Design review of the part built by this model. Coordinates are the model's own, in mm. A direction names the side the tool comes from. Round coordinates to 2 decimals unless told otherwise and drop trailing zeros. Loops run counter-clockwise (first coordinate to the right, second up) from the corner with the lowest first, then second, coordinate; pieces in that order, holes last. Notation, with made-up numbers: (51.25, -24) - (60.25, -24) arc R12 cw to (60.25, -6) - close; hole circle Ø2 at (25, 34.25). An arc over 180 degrees is marked (long way). Answer as CSV lines item,"result". Start each with the question number.
(1) Consider section B-B (y = 0). Count the separate pieces of the cut face and the enclosed holes in it, and give its area (3 significant figures).
(2) For P1, Ø1, axis at x = 140.5, z = 4.5, coming from the -Y side; P2, Ø12, axis at x = 28.5, y = 2, coming from the -Z side; P3, Ø6, axis at y = 10, z = -6, coming from the -X side, all flat-tipped, find the tip position at first contact; note any pin that passes through.
(3) Consider section C-C (z = 22). Give the boundary of the cut face in (x, y).
(4) Consider section A-A (x = 0). Give the boundary of the cut face in (y, z), and give its area (3 significant figures).
(5) For faces 3 (the flat face through (-3, -5.4, 0)), 4 (the cylindrical face through (132.387, 7.154, 2.253)), 5 (the flat face through (-3, -5.4, 25)), list the 3-axis set-ups (+Z, -Z, +X, -X, +Y, -Y) from which the entire face can be reached by the end or side of a thin tool; tool diameter is ignored.
(6) Mouldability with a two-part tool opening along X and no side actions: class faces 1 (the cylindrical face through (161.923, 3.755, 0.175)), 2 (the flat face through (155.4, 3, 12.5)) as released by +X, released by -X, zero draft, split by the parting line, or undercut.
(7) Wall thickness on L1, parallel to Y at x = 150, z = 0; L2, parallel to Z at x = -4.5, y = -8; L3, parallel to Y at x = 51, z = 9: over which ranges is each line inside the solid? List them lowest first.
from build123d import *

# Parameters (mm, degrees)
F0_R      = 12.5
F0_R_2    = 6
F1_DEPTH  = 25
F3_R      = 12.5
F3_R_2    = 6
F4_DEPTH  = 12.5
F5_R      = 7.5
F7_R      = 6
F8_DEPTH  = 25
F9_R      = 6
F10_DEPTH = 25


# Not quite as in the source:
# - a feature names something its author has since deleted; it is built from what else it names


with BuildPart() as f1:
    # F0 (on Top) → F1 (new body)
    with BuildSketch(Plane.XY):
        Circle(F0_R)
        Circle(F0_R_2, mode=Mode.SUBTRACT)
    extrude(amount=F1_DEPTH)



with BuildPart() as f4:
    # F3 (on Top) → F4 (new body, symmetric)
    with BuildSketch(Plane.XY):
        with Locations((150, 0)):
            Circle(F3_R)
        with Locations((150, 0)):
            Circle(F3_R_2, mode=Mode.SUBTRACT)
    extrude(amount=F4_DEPTH, both=True)


with BuildPart() as f1_1:
    add(f1.part)

    add(f4.part)  # F6 merges F4
    # F6: sweep along a path in F2
    with BuildLine(Plane.XZ) as f6_path:
        Line((0, 12.5), (25, 12.5))
        ThreePointArc((25, 12.5), (33.2790451747, 11.9260667636), (41.399703043, 10.2152470332))
        Line((41.399703043, 10.2152470332), (64.3324330449, 6.6001820378))
        Line((64.3324330449, 6.6001820378), (81.3044384122, 4.0990444832))
        Line((81.3044384122, 4.0990444832), (108.4596440196, 1.9552123267))
        Line((108.4596440196, 1.9552123267), (125, 0))
        Line((125, 0), (150, 0))
    # F5 (on Right) → F6 (sweep)
    with BuildSketch(Plane.YZ):
        with Locations((0, 12.5)):
            Circle(F5_R)
    sweep(path=f6_path.line, transition=Transition.RIGHT)

    # F7 (on Top) → F8 (cut)
    with BuildSketch(Plane.XY):
        Circle(F7_R)
    extrude(amount=F8_DEPTH, mode=Mode.SUBTRACT)

    # F9 (on face) → F10 (cut)
    with BuildSketch(Plane.XY.offset(12.5)):
        with Locations((150, 0)):
            Circle(F9_R)
    extrude(amount=-F10_DEPTH, mode=Mode.SUBTRACT)


solid = f1_1.part
Determined:
1,separate pieces,"3"
1,enclosed holes,"0"
1,area,"2,540 mm^2"
2,P1,"stops at y = -8.67"
2,P2,"stops at z = 4.18"
2,P3,"stops at x = 139.64"
3,outline,"circle Ø25 at (0, 0); hole circle Ø12 at (0, 0)"
4,outline,"(-12.5, 0) - (-6, 0) - (-6, 25) - (-12.5, 25) - close; (6, 0) - (12.5, 0) - (12.5, 25) - (6, 25) - close"
4,area,"325 mm^2"
5,face 3,"-Z, -X, +Y, -Y"
5,face 4,"none"
5,face 5,"+Z, +X, -X, +Y, -Y"
6,face 1,"undercut"
6,face 2,"zero draft"
7,L1,"y = -12.5 to -6, 6 to 12.5"
7,L2,"z = 0 to 25"
7,L3,"y = -7.49 to 7.49"
